```python
from build123d import *

# Parameters (mm, degrees)
BOSS_EXTRUDE1_DEPTH = 4
SKETCH2_R           = 1.5
BOSS_EXTRUDE2_DEPTH = 3
CUT_EXTRUDE1_DEPTH  = 13
CUT_EXTRUDE2_DEPTH  = 49
CUT_EXTRUDE3_DEPTH  = 37
SKETCH6_R           = 1.5
BOSS_EXTRUDE3_DEPTH = 5
SKETCH7_W           = 11
SKETCH7_H           = 1
CUT_EXTRUDE4_DEPTH  = 2
CUT_EXTRUDE5_START  = -12
SKETCH7_2_W         = 11
SKETCH7_2_H         = 1
CUT_EXTRUDE5_DEPTH  = 2
SKETCH8_W           = 14
SKETCH8_H           = 4
BOSS_EXTRUDE4_DEPTH = 3
SKETCH9_W           = 5
SKETCH9_H           = 4
BOSS_EXTRUDE5_DEPTH = 12
CUT_EXTRUDE6_DEPTH  = 4.5
CUT_EXTRUDE7_START  = -14
CUT_EXTRUDE7_DEPTH  = 4.5


with BuildPart() as part:
    # Sketch1 → Boss-Extrude1 (new body)
    with BuildSketch(Plane(origin=(0, 0, 0), x_dir=(1, 0, 0), z_dir=(0, 1, 0))):
        Polygon((-1, 15), (2, 15), (18, 7), (23, 7), (23, -7), (18, -7), (2, -15), (-1, -15), (-7, -6), (-42, -6), (-42, 6), (-7, 6), align=None)
    extrude(amount=BOSS_EXTRUDE1_DEPTH)

    # Sketch2 → Boss-Extrude2 (add)
    with BuildSketch(Plane(origin=(0, 4, 0), x_dir=(1, 0, 0), z_dir=(0, 1, 0))):
        with Locations(Location((-1.5, 8, 0), (0, 0, 270))):
            Circle(SKETCH2_R)
        with Locations(Location((-1.5, -8, 0), (0, 0, 90))):
            Circle(SKETCH2_R)
    extrude(amount=BOSS_EXTRUDE2_DEPTH)

    # Sketch3 → Cut-Extrude1 (cut)
    with BuildSketch(Plane.XY.offset(6)):
        Polygon((-24, 0), (-42, 2), (-42, 0), align=None)
    extrude(amount=-CUT_EXTRUDE1_DEPTH, mode=Mode.SUBTRACT)

    # Sketch4 → Cut-Extrude2 (cut, along a direction that is not the sketch's normal)
    with BuildSketch(Plane.ZY.offset(42)):
        with BuildLine():
            ThreePointArc((-5, 2), (-5.736067977, 2.881966011), (-6, 4))
            Line((-6, 4), (-6, 2))
            Line((-6, 2), (-5, 2))
        make_face()
        with BuildLine():
            Line((1.25, 2.910275264), (-1.25, 2.910275264))
            ThreePointArc((-1.25, 2.910275264), (-1.570550528, 2.410275264), (-2, 2))
            Line((-2, 2), (2, 2))
            ThreePointArc((2, 2), (1.570550528, 2.410275264), (1.25, 2.910275264))
        make_face()
        with BuildLine():
            Line((5, 2), (6, 2))
            Line((6, 2), (6, 4))
            ThreePointArc((6, 4), (5.736067977, 2.881966011), (5, 2))
        make_face()
    extrude(amount=-CUT_EXTRUDE2_DEPTH, dir=(-0.9938837346736189, 0.11043152607484653, 0), mode=Mode.SUBTRACT)

    # Sketch5 → Cut-Extrude3 (cut)
    with BuildSketch(Plane.XY.offset(15)):
        Polygon((-7, 4), (8, 4), (8, 2.5), (-7, 2.5), (-16, 2.5), (-16, 4), align=None)
    extrude(amount=-CUT_EXTRUDE3_DEPTH, mode=Mode.SUBTRACT)


with BuildPart() as cut_extrude3_piece_1:
    # of the separate pieces the step leaves, piece 1, a body of its own (cut_extrude3_pieces)
    add(part.part.solids().sort_by_distance((-1, 0, -15))[0])



with BuildPart() as cut_extrude3_piece_2:
    # of the separate pieces the step leaves, piece 2, a body of its own (cut_extrude3_pieces)
    add(part.part.solids().sort_by_distance((-1.5, 4, -6.5))[0])


with BuildPart() as cut_extrude3_piece_3:
    # of the separate pieces the step leaves, piece 3, a body of its own (cut_extrude3_pieces)
    add(part.part.solids().sort_by_distance((-1.5, 4, 6.5))[0])


with BuildPart() as cut_extrude3_piece_1_1:
    add(cut_extrude3_piece_1.part)

    add(cut_extrude3_piece_2.part)  # Boss-Extrude3 merges Cut-Extrude3 piece 2

    add(cut_extrude3_piece_3.part)  # Boss-Extrude3 merges Cut-Extrude3 piece 3
    # Sketch6 → Boss-Extrude3 (add)
    with BuildSketch(Plane(origin=(0, 7, 0), x_dir=(1, 0, 0), z_dir=(0, 1, 0))):
        with Locations(Location((-1.5, -8, 0), (0, 0, 270))):
            Circle(SKETCH6_R)
        with Locations(Location((-1.5, 8, 0), (0, 0, 270))):
            Circle(SKETCH6_R)
    extrude(amount=-BOSS_EXTRUDE3_DEPTH)

    # Sketch7 → Cut-Extrude4 (cut)
    with BuildSketch(Plane.XY.offset(6)):
        with Locations((-34, 3.5)):
            Rectangle(SKETCH7_W, SKETCH7_H)
    extrude(amount=-CUT_EXTRUDE4_DEPTH, mode=Mode.SUBTRACT)

    # Sketch7<2> → Cut-Extrude5 (cut)
    with BuildSketch(Plane.XY.offset(6).offset(CUT_EXTRUDE5_START)):
        with Locations((-34, 3.5)):
            Rectangle(SKETCH7_2_W, SKETCH7_2_H)
    extrude(amount=CUT_EXTRUDE5_DEPTH, mode=Mode.SUBTRACT)

    # Sketch8 → Boss-Extrude4 (add)
    with BuildSketch(Plane(origin=(23, 0, 0), x_dir=(0, 0, -1), z_dir=(1, 0, 0))):
        with Locations((0, 2)):
            Rectangle(SKETCH8_W, SKETCH8_H)
    extrude(amount=BOSS_EXTRUDE4_DEPTH)

    # Sketch9 → Boss-Extrude5 (add)
    with BuildSketch(Plane(origin=(26, 0, 0), x_dir=(0, 0, -1), z_dir=(1, 0, 0))):
        with Locations((0, 2)):
            Rectangle(SKETCH9_W, SKETCH9_H)
    extrude(amount=BOSS_EXTRUDE5_DEPTH)

    # Sketch10 → Cut-Extrude6 (cut)
    with BuildSketch(Plane.XY.offset(7)):
        Polygon((18, 0), (22, 4), (26, 4), (26, 0), align=None)
    extrude(amount=-CUT_EXTRUDE6_DEPTH, mode=Mode.SUBTRACT)

    # Sketch10<3> → Cut-Extrude7 (cut)
    with BuildSketch(Plane.XY.offset(7).offset(CUT_EXTRUDE7_START)):
        Polygon((18, 0), (22, 4), (26, 4), (26, 0), align=None)
    extrude(amount=CUT_EXTRUDE7_DEPTH, mode=Mode.SUBTRACT)


solid = cut_extrude3_piece_1_1.part
```
CAD build for the part. Positions are in the model's coordinates, mm. A direction names the side the tool comes from. Round coordinates to 2 decimals unless told otherwise and drop trailing zeros. Order: outer loops, then holes, each group sorted by start corner. A loop starts at its lowest first (then second) coordinate and runs counter-clockwise, first axis right, second up. Notation, with made-up numbers: (16.5, -1) - (48.5, -1) arc R16 cw to (48.5, 25) - close; hole circle Ø5 at (9.5, 43). An arc over 180 degrees is marked (long way). Answer as CSV lines item,"result". Start each with the question number.
1. Saw through at B-B, the plane x = 16.5. Write the cut outline in (y, z).
2. Saw through at A-A, the plane z = 8. Write the cut outline in (x, y).
3. Pull direction X, two halves, no side cores. Call faces 6 (the face through (19, 3, 7)), 7 (the face through (-29.087, 1.476, 0.017)), 8 (the face through (-2, 2.5, 0)): +X half, -X half, draft (parallel to the pull), parting line (faces both ways), or undercut.
4. Drill centre lines: L1, parallel to X at y = 3.5, z = 1; L2, parallel to Y at x = 11.5, z = -5; L3, parallel to Y at x = 7, z = 4. Where is each one in solid material? Low to high. Write a range as [from, to].
5. Tool access for faces 1 (the face through (19, 3, -7)), 2 (the face through (-1.43, 4.78, -9.5)), 3 (the face through (19, 4, 0)), 4 (the face through (-17, 2, 6)), 5 (the face through (28, 2, 2.5)): list every direction of +Z, -Z, +X, -X, +Y, -Y with a clear straight run to the whole face (end or side of a thin tool).
6. Pin check, flat tips, straight feed: pin 1 (0.5 mm diameter, centred on x = -31.5, y = 3.5, fed in from -Z); pin 2 (6 mm diameter, centred on x = -8.5, z = 7, fed in from +Y); pin 3 (1.2 mm diameter, centred on x = 25.5, y = 2, fed in from +Z); pin 4 (10 mm diameter, centred on x = 3.5, z = 5, fed in from +Y). Stop position of each tip, or through.
7. Saw through at C-C, the plane x = 32.5. Write the cut outline in (y, z), and give its area (3 significant figures).
Model answer:
1,outline,"(0, -7.75) - (4, -7.75) - (4, 7.75) - (0, 7.75) - close"
2,outline,"(-5.67, 0) - (16, 0) - (16, 4) - (8, 4) - (8, 2.5) - (0, 2.5) - (0, 7) - (-3, 7) - (-3, 2.5) - (-5.67, 2.5) - close"
3,face 6,"draft"
3,face 7,"-X half"
3,face 8,"undercut"
4,L1,"x = [-42, -16], [8, 38]"
4,L2,"y = [0, 4]"
4,L3,"y = [0, 2.5]"
5,face 1,"-Z, +X, +Y, -Y"
5,face 2,"+Y"
5,face 3,"+Z, -Z, +X, +Y"
5,face 4,"+Z, -X, +Y, -Y"
5,face 5,"+Z, +X, -Y"
6,pin 1,"stops at z = -4"
6,pin 2,"stops at y = 2.5"
6,pin 3,"stops at z = 2.5"
6,pin 4,"stops at y = 7"
7,outline,"(0, -2.5) - (4, -2.5) - (4, 2.5) - (0, 2.5) - close"
7,area,"20.0 mm²"
